CAD build for the part. Positions are in the model's coordinates, mm. Coordinates: 2 decimals unless noted, no trailing zeros. Order: outer loops, then holes, each group sorted by start corner. A loop starts at its lowest first (then second) coordinate and runs counter-clockwise, first axis right, second up. Notation, with made-up numbers: (-17, 73) - (-7, 73) arc R8 ccw to (-7, 82) - close; hole circle Ø6 at (-11.75, 15). An arc over 180 degrees is marked (long way). Return JSON: item names as keys, results as strings.
from build123d import *

# Parameters (mm, degrees)
BOSS_EXTRUDE1_DEPTH = 3


with BuildPart() as part:
    # Sketch1 → Boss-Extrude1 (new body)
    with BuildSketch(Plane.XY):
        with BuildLine():
            Line((-173.5, 0), (173.5, 0))
            Line((173.5, 0), (173.5, -80))
            ThreePointArc((173.5, -80), (170.571067812, -87.071067812), (163.5, -90))
            Line((163.5, -90), (133.5, -90))
            ThreePointArc((133.5, -90), (126.428932188, -87.071067812), (123.5, -80))
            Line((123.5, -80), (123.5, -75))
            ThreePointArc((123.5, -75), (122.035533906, -71.464466094), (118.5, -70))
            Line((118.5, -70), (-118.5, -70))
            ThreePointArc((-118.5, -70), (-122.035533906, -71.464466094), (-123.5, -75))
            Line((-123.5, -75), (-123.5, -80))
            ThreePointArc((-123.5, -80), (-126.428932188, -87.071067812), (-133.5, -90))
            Line((-133.5, -90), (-163.5, -90))
            ThreePointArc((-163.5, -90), (-170.571067812, -87.071067812), (-173.5, -80))
            Line((-173.5, -80), (-173.5, 0))
        make_face()
        with BuildLine():
            Line((36, -7.5), (136, -7.5))
            ThreePointArc((136, -7.5), (138.5, -10), (136, -12.5))
            Line((136, -12.5), (36, -12.5))
            ThreePointArc((36, -12.5), (33.5, -10), (36, -7.5))
        make_face(mode=Mode.SUBTRACT)
        with BuildLine():
            Line((-36, -7.5), (-136, -7.5))
            ThreePointArc((-136, -7.5), (-138.5, -10), (-136, -12.5))
            Line((-136, -12.5), (-36, -12.5))
            ThreePointArc((-36, -12.5), (-33.5, -10), (-36, -7.5))
        make_face(mode=Mode.SUBTRACT)
    extrude(amount=BOSS_EXTRUDE1_DEPTH)


solid = part.part
Item 1: Band-saw the part on A-A, the plane x = -39.5. List the corners of the cut face in (y, z), then the cut area to 3 significant figures.
Findings below:
{"outline": "(-70, 0) - (-12.5, 0) - (-12.5, 3) - (-70, 3) - close; (-7.5, 0) - (0, 0) - (0, 3) - (-7.5, 3) - close", "area": "195 mm²"}
Item 2: Drop a flat-ended pin along its axis: P1, Ø1.5, axis at x = -42.5, z = 1, coming from the -Y side. Give the stop position or say it passes through.
Findings below:
{"P1": "stops at y = -70"}
Item 3: Wall check: L1, parallel to Y at x = -41, z = 1.1; L2, parallel to X at y = -75, z = 2.75; L3, parallel to X at y = -70.5, z = 1.55. Give the ranges that are in metal, low to high. Write a range as [from, to].
Findings below:
{"L1": "y = [-70, -12.5], [-7.5, 0]", "L2": "x = [-173.5, -123.5], [123.5, 173.5]", "L3": "x = [-173.5, -120.68], [120.68, 173.5]"}
Item 4: Band-saw the part on B-B, the plane z = 1.2. List the corners of the cut face in (x, y).
Findings below:
{"outline": "(-173.5, -80) arc R10 ccw to (-163.5, -90) - (-133.5, -90) arc R10 ccw to (-123.5, -80) - (-123.5, -75) arc R5 cw to (-118.5, -70) - (118.5, -70) arc R5 cw to (123.5, -75) - (123.5, -80) arc R10 ccw to (133.5, -90) - (163.5, -90) arc R10 ccw to (173.5, -80) - (173.5, 0) - (-173.5, 0) - close; hole (-136, -12.5) - (-36, -12.5) arc R2.5 ccw to (-36, -7.5) - (-136, -7.5) arc R2.5 ccw to start; hole (36, -12.5) - (136, -12.5) arc R2.5 ccw to (136, -7.5) - (36, -7.5) arc R2.5 ccw to start"}
Item 5: Band-saw the part on C-C, the plane x = -0.5. List the corners of the cut face in (y, z), then the cut area to 3 significant figures.
Findings below:
{"outline": "(-70, 0) - (0, 0) - (0, 3) - (-70, 3) - close", "area": "210 mm²"}
Item 6: Mould opens along X. For faces 1 (the cylindrical face through (170.65, -86.99, 1.48)), 2 (the flat face through (2, -34, 3)), 3 (the cylindrical face through (126.51, -87.15, 1.48)), 4 (the cylindrical face through (-126.35, -86.99, 1.48)) say: released by +X, released by -X, zero draft, split by the parting line, or undercut.
Findings below:
{"face 1": "released by +X", "face 2": "zero draft", "face 3": "undercut", "face 4": "undercut"}
